Design review of the part built by this model. Coordinates are the model's own, in mm. Coordinates: 2 decimals unless noted, no trailing zeros. Loops run counter-clockwise (first coordinate to the right, second up) from the corner with the lowest first, then second, coordinate; pieces in that order, holes last. Notation, with made-up numbers: (-33.5, 59.25) -> (-19.5, 59.25) arc R26 ccw to (-19.5, 73.25) -> close; hole circle Ø10 at (-1, 41). An arc over 180 degrees is marked (long way). One line per item, written item: value. Start each with the question number.
1. Add section A-A on z = 4. Write out the cut boundary in (x, y) (1 decimal), plus the area to 3 significant figures.
2. Add section D-D on z = 10. Write out the cut boundary in (x, y) (3 decimals).
3. For probe 1 along X at (y, z) = (0.2, 2.5); probe 2 along Z at (x, y) = (42.5, 1.95); probe 3 along X at (y, z) = (3, 1.5), list the stretches that pass through material, from the lowest coordinate up.
4. Insertion check: pin 1 (1.6 mm diameter, centred on x = 0.5, y = 1.5, fed in from -Z); pin 2 (1.6 mm diameter, centred on y = 2, z = 4, fed in from -X); pin 3 (1.6 mm diameter, centred on y = 2, z = -2.5, fed in from -X); pin 4 (4 mm diameter, centred on x = 37.5, z = 16, fed in from +Y). Each pin has a flat end and moves straight along its axis. Give the tip position at first contact, or say it passes through.
5. Add section B-B on x = 12. Write out the cut boundary in (y, z) (3 decimals).
6. Add section C-C on z = 15.5. Write out the cut boundary in (x, y) (3 decimals).
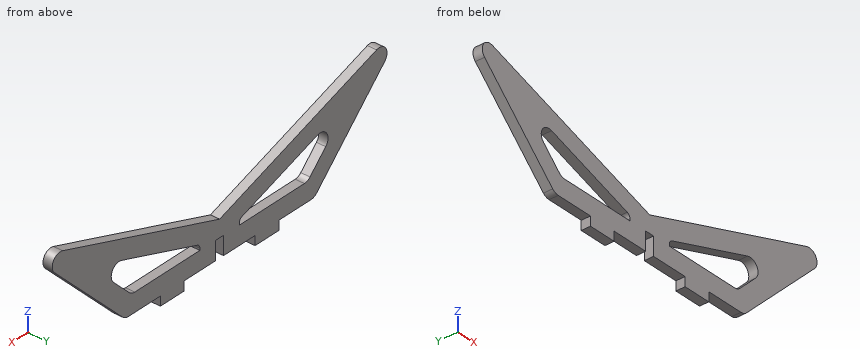
```python
from build123d import *

# Parameters (mm, degrees)
BOSS_EXTRUDE1_DEPTH = 3.175


with BuildPart() as part:
    # Sketch1 → Boss-Extrude1 (new body)
    with BuildSketch(Plane(origin=(0, 0, 0), x_dir=(1, 0, 0), z_dir=(0, 1, 0))):
        with BuildLine():
            Line((-36.784871939, 0), (-23.8125, 0))
            Line((-23.8125, 0), (-23.8125, 3.175))
            Line((-23.8125, 3.175), (-14.2875, 3.175))
            Line((-14.2875, 3.175), (-14.2875, 0))
            Line((-14.2875, 0), (-1.5875, 0))
            Line((-1.5875, 0), (-1.5875, -6.35))
            Line((-1.5875, -6.35), (1.5875, -6.35))
            Line((1.5875, -6.35), (1.5875, 0))
            Line((1.5875, 0), (14.2875, 0))
            Line((14.2875, 0), (14.2875, 3.175))
            Line((14.2875, 3.175), (23.8125, 3.175))
            Line((23.8125, 3.175), (23.8125, 0))
            Line((23.8125, 0), (36.784871939, 0))
            ThreePointArc((36.784871939, 0), (37.999891837, -0.241682484), (39.02993597, -0.92993597))
            Line((39.02993597, -0.92993597), (66.469065694, -28.369065694))
            ThreePointArc((66.469065694, -28.369065694), (66.920159512, -32.290840151), (63.203219493, -33.620560958))
            Line((63.203219493, -33.620560958), (0, -12.160991598))
            Line((0, -12.160991598), (-63.203219493, -33.620560958))
            ThreePointArc((-63.203219493, -33.620560958), (-66.920159512, -32.290840151), (-66.469065694, -28.369065694))
            Line((-66.469065694, -28.369065694), (-39.02993597, -0.92993597))
            ThreePointArc((-39.02993597, -0.92993597), (-37.999891837, -0.241682484), (-36.784871939, 0))
        make_face()
        with BuildLine():
            Line((-39.452913677, -18.850511262), (-9.014608915, -8.515706841))
            ThreePointArc((-9.014608915, -8.515706841), (-8.234573307, -7.9371291), (-7.9375, -7.012491225))
            Line((-7.9375, -7.012491225), (-7.9375, -6.35))
            Line((-7.9375, -6.35), (-34.154615818, -6.35))
            ThreePointArc((-34.154615818, -6.35), (-35.369635716, -6.591682484), (-36.399679849, -7.27993597))
            Line((-36.399679849, -7.27993597), (-42.718759878, -13.599015999))
            ThreePointArc((-42.718759878, -13.599015999), (-43.169853696, -17.520790456), (-39.452913677, -18.850511262))
        make_face(mode=Mode.SUBTRACT)
        with BuildLine():
            Line((39.452913677, -18.850511262), (9.014608915, -8.515706841))
            ThreePointArc((9.014608915, -8.515706841), (8.234573307, -7.9371291), (7.9375, -7.012491225))
            Line((7.9375, -7.012491225), (7.9375, -6.35))
            Line((7.9375, -6.35), (34.154615818, -6.35))
            ThreePointArc((34.154615818, -6.35), (35.369635716, -6.591682484), (36.399679849, -7.27993597))
            Line((36.399679849, -7.27993597), (42.718759878, -13.599015999))
            ThreePointArc((42.718759878, -13.599015999), (43.169853696, -17.520790456), (39.452913677, -18.850511262))
        make_face(mode=Mode.SUBTRACT)
    extrude(amount=BOSS_EXTRUDE1_DEPTH)


solid = part.part
```
Worked answers:
1. outline: (-42.1, 0) -> (-1.6, 0) -> (-1.6, 3.2) -> (-42.1, 3.2) -> close; (1.6, 0) -> (42.1, 0) -> (42.1, 3.2) -> (1.6, 3.2) -> close
1. area: 257 mm²
2. outline: (-48.1, 0) -> (-39.12, 0) -> (-39.12, 3.175) -> (-48.1, 3.175) -> close; (-13.386, 0) -> (13.386, 0) -> (13.386, 3.175) -> (-13.386, 3.175) -> close; (39.12, 0) -> (48.1, 0) -> (48.1, 3.175) -> (39.12, 3.175) -> close
3. probe 1: x = -40.6 to -1.59, 1.59 to 40.6
3. probe 2: z = 4.4 to 13.38, 18.29 to 26.59
3. probe 3: x = -39.6 to -1.59, 1.59 to 39.6
4. pin 1: stops at z = 6.35
4. pin 2: stops at x = -42.9
4. pin 3: stops at x = -23.81
4. pin 4: passes through
5. outline: (0, 0) -> (3.175, 0) -> (3.175, 6.35) -> (0, 6.35) -> close; (0, 9.529) -> (3.175, 9.529) -> (3.175, 16.235) -> (0, 16.235) -> close
6. outline: (-53.6, 0) -> (-43.63, 0) -> (-43.63, 3.175) -> (-53.6, 3.175) -> close; (-29.585, 0) -> (-9.834, 0) -> (-9.834, 3.175) -> (-29.585, 3.175) -> close; (9.834, 0) -> (29.585, 0) -> (29.585, 3.175) -> (9.834, 3.175) -> close; (43.63, 0) -> (53.6, 0) -> (53.6, 3.175) -> (43.63, 3.175) -> close
